For this review, take the finished solid that the model builds, in its own axes (mm). Give positions to 0.01 mm unless a question says otherwise; leave off trailing zeros. Write each loop counter-clockwise with the first axis right and the second up, starting at its lowest first coordinate (ties: lowest second). Pieces come first, ordered by that corner, then holes. Notation, with made-up numbers: M -32.5,-38.75 L 13.5,-38.75 A18 ccw 13.5,-22.75 Z; hole C -5.5,-15.75 d3. An arc over 180 degrees is marked long. Answer as a JSON object with one key per item and string values. Group by question number.
```python
from build123d import *

# Parameters (mm, degrees)
SKETCH_1_R      = 1.5
EXTRUDE_1_DEPTH = 4


with BuildPart() as part:
    # 草图1 → 凸台-拉伸1 (new body)
    with BuildSketch(Plane.XY):
        Polygon((0, 0), (0, 94), (-55.5, 94), (-93, 20), (-93, 0), (-60.5, -46), (-40.5, -46), align=None)
        with Locations((-86.5, 15)):
            Circle(SKETCH_1_R, mode=Mode.SUBTRACT)
        with Locations(Location((-86.5, 5, 0), (0, 0, 180))):
            Circle(SKETCH_1_R, mode=Mode.SUBTRACT)
        with Locations((-6.5, 5)):
            Circle(SKETCH_1_R, mode=Mode.SUBTRACT)
        with Locations(Location((-6.5, 15, 0), (0, 0, 180))):
            Circle(SKETCH_1_R, mode=Mode.SUBTRACT)
        with Locations((-25.5, 80)):
            Circle(SKETCH_1_R, mode=Mode.SUBTRACT)
        with Locations((-25.5, 70)):
            Circle(SKETCH_1_R, mode=Mode.SUBTRACT)
        with Locations((-50.5, 10)):
            Circle(SKETCH_1_R, mode=Mode.SUBTRACT)
        with Locations((-50.5, 30)):
            Circle(SKETCH_1_R, mode=Mode.SUBTRACT)
        with Locations((-50.5, 50)):
            Circle(SKETCH_1_R, mode=Mode.SUBTRACT)
        with Locations((-50.5, -10)):
            Circle(SKETCH_1_R, mode=Mode.SUBTRACT)
        with Locations((-50.5, -30)):
            Circle(SKETCH_1_R, mode=Mode.SUBTRACT)
        with Locations((-5, 88)):
            Circle(SKETCH_1_R, mode=Mode.SUBTRACT)
        with Locations((-25, 88)):
            Circle(SKETCH_1_R, mode=Mode.SUBTRACT)
        with Locations((-50.5, 70)):
            Circle(SKETCH_1_R, mode=Mode.SUBTRACT)
    extrude(amount=EXTRUDE_1_DEPTH)


solid = part.part
```
Item 1: Consider section A-A (x = -50.5). Give the boundary of the cut face in (y, z), plus the area to 3 significant figures.
Item 2: Consider section C-C (y = 80). Give the boundary of the cut face in (x, z), plus the area to 3 significant figures.
Item 3: Consider section D-D (x = -86.5). Give the boundary of the cut face in (y, z).
Item 4: Insertion check: P1, Ø2.5, axis at x = -25.5, y = 80, coming from the +Z side; P2, Ø1, axis at y = -17.5, z = 0.5, coming from the -X side; P3, Ø2, axis at x = -65, z = 1.5, coming from the -Y side. Each pin has a flat end and moves straight along its axis. Give the tip position at first contact, or say it passes through.
Item 5: To check wall thickness, follow probe 1 along Y at (x, z) = (-87.5, 3.5); probe 2 along Y at (x, z) = (-7, 1.75); probe 3 along X at (y, z) = (80, 2.95). State the ranges of each line that lie inside material, in increasing order.
Item 6: Consider section B-B (z = 3.35). State how many separate pieces and enclosed holes the cut face has, plus the area to 3 significant figures.
Item 7: Draft analysis for pull direction X (two halves, no side actions). For faces 1 (the flat face through (-76.977, -22.678, 1.972)), 2 (the cylindrical face through (-25.695, 71.487, 1.972)), 3 (the flat face through (0, 46, 2)), state which applies: released by +X, released by -X, zero draft, split by the parting line, or undercut.
Result set:
{
 "1": {"outline": "M -46,0 L -31.5,0 L -31.5,4 L -46,4 Z; M -28.5,0 L -11.5,0 L -11.5,4 L -28.5,4 Z; M -8.5,0 L 8.5,0 L 8.5,4 L -8.5,4 Z; M 11.5,0 L 28.5,0 L 28.5,4 L 11.5,4 Z; M 31.5,0 L 48.5,0 L 48.5,4 L 31.5,4 Z; M 51.5,0 L 68.5,0 L 68.5,4 L 51.5,4 Z; M 71.5,0 L 94,0 L 94,4 L 71.5,4 Z", "area": "488 mm^2"},
 "2": {"outline": "M -62.59,0 L -27,0 L -27,4 L -62.59,4 Z; M -24,0 L 0,0 L 0,4 L -24,4 Z", "area": "238 mm^2"},
 "3": {"outline": "M -9.2,0 L 3.5,0 L 3.5,4 L -9.2,4 Z; M 6.5,0 L 13.5,0 L 13.5,4 L 6.5,4 Z; M 16.5,0 L 32.83,0 L 32.83,4 L 16.5,4 Z"},
 "4": {"P1": "passes through", "P2": "stops at x = -80.99", "P3": "stops at y = -41.05"},
 "5": {"probe 1": "y = -7.78 to 3.88, 6.12 to 13.88, 16.12 to 30.85", "probe 2": "y = -7.95 to 3.59, 6.41 to 13.59, 16.41 to 94", "probe 3": "x = -62.59 to -27, -24 to 0"},
 "6": {"separate pieces": "1", "enclosed holes": "14", "area": "9,850 mm^2"},
 "7": {"face 1": "released by -X", "face 2": "undercut", "face 3": "released by +X"}
}
